Here's how the part is built. I have some questions about the finished solid (model axes, mm). A direction names the side the tool comes from. Round coordinates to 2 decimals unless told otherwise and drop trailing zeros. Order: outer loops, then holes, each group sorted by start corner. A loop starts at its lowest first (then second) coordinate and runs counter-clockwise, first axis right, second up. Notation, with made-up numbers: (50, 22.25) - (89, 22.25) arc R16 ccw to (89, 40.25) - close; hole circle Ø11 at (73, 46.25). An arc over 180 degrees is marked (long way). Answer as a JSON object with one key per item and string values.
```python
from build123d import *

# Parameters (mm, degrees)
BOSS_EXTRUDE1_DEPTH     = 7.14375
SKETCH2_R               = 4.5
CUT_EXTRUDE1_DEPTH      = 31.286531402
CUT_EXTRUDE2_REACH      = 26.287
CUT_EXTRUDE2_END_RADIUS = 4.5
SKETCH3_R               = 4.5


with BuildPart() as part:
    # Sketch1 → Boss-Extrude1 (new, symmetric)
    with BuildSketch(Plane(origin=(0, 0, 0), x_dir=(0, 0, -1), z_dir=(1, 0, 0))):
        Polygon((-13.49375, -7.14375), (13.49375, -7.14375), (13.49375, 7.14375), (7.14375, 7.14375), (7.14375, 11.74375), (-7.14375, 11.74375), (-7.14375, 7.14375), (-13.49375, 7.14375), align=None)
    extrude(amount=BOSS_EXTRUDE1_DEPTH, both=True)

    # Sketch2 → Cut-Extrude1 (cut, through all)
    with BuildSketch(Plane.XY.offset(13.49375)):
        Circle(SKETCH2_R)
    extrude(amount=-CUT_EXTRUDE1_DEPTH, mode=Mode.SUBTRACT)

    # Cut-Extrude2: up to this cylinder (the profile starts outside it)
    cut_extrude2_end = Plane(origin=(0, 0, 0), z_dir=(0, 0, 1)) * Cylinder(CUT_EXTRUDE2_END_RADIUS, 62.574, mode=Mode.PRIVATE)
    # Sketch3 → Cut-Extrude2 (cut, up to the surface)
    with BuildSketch(Plane(origin=(0, 11.74375, 0), x_dir=(1, 0, 0), z_dir=(0, 1, 0)), mode=Mode.PRIVATE) as cut_extrude2_sk1:
        with Locations(Location((0, 0, 0), (0, 0, 270))):
            Circle(SKETCH3_R)
    cut_extrude2_tool1 = extrude(cut_extrude2_sk1.sketch, amount=-CUT_EXTRUDE2_REACH, mode=Mode.PRIVATE) - cut_extrude2_end
    add(cut_extrude2_tool1.solids().sort_by_distance((0, 11.74375, 0))[0], mode=Mode.SUBTRACT)

    # Sketch4 → Cut-Revolve1 (revolve, cut)
    with BuildSketch(Plane(origin=(0, 0, 0), x_dir=(0, 0, -1), z_dir=(0.7071067811865476, 0.7071067811865475, 0))):
        Polygon((13.49375, 10.102788136), (13.99375, 6.967405384), (11.90625, 10.102788136), align=None)
        Polygon((-13.49375, 10.102788136), (-13.99375, 6.967405384), (-11.90625, 10.102788136), align=None)
    revolve(axis=Axis((0, 0, -13.49375), (0, 0, 1)), mode=Mode.SUBTRACT)

    # Sketch5 → Cut-Revolve2 (revolve, cut)
    with BuildSketch(Plane(origin=(0, 0, 0), x_dir=(-0.7071067811865476, 0, -0.7071067811865475), z_dir=(0.7071067811865475, 0, -0.7071067811865476))):
        Polygon((10.102788136, 11.74375), (6.967405384, 12.24375), (10.102788136, 10.15625), align=None)
    revolve(axis=Axis((0, 0, 0), (0, 1, 0)), mode=Mode.SUBTRACT)


solid = part.part
```
1. For faces 1 (the face through (0, 9, -7.144)), 2 (the face through (3.3, 11.744, -3.3)), which set-ups out of +Z, -Z, +X, -X, +Y, -Y let a thin tool reach every point of the face, with its end or its side?
Responses:
{"face 1": "-Z, +X, -X, +Y", "face 2": "+Z, -Z, +X, -X, +Y"}
2. Thinking about a two-plate mould opening in Z: for faces 3 (the face through (5.971, 5.905, -13.042)), 4 (the face through (4.46, 7.26, -0.59)), 5 (the face through (0, 9, 7.144)), which applies, pulls with the +Z half, pulls with the -Z half, needs draft (parallel to the pull), parting line crosses it, or undercut?
Responses:
{"face 3": "pulls with the -Z half", "face 4": "undercut", "face 5": "pulls with the +Z half"}
3. Imagine slicing it at B-B (y = 8). List the corners of the cut face in (x, z) for me, plus the area to 3 significant figures.
Responses:
{"outline": "(-7.14, -7.14) - (7.14, -7.14) - (7.14, 7.14) - (-7.14, 7.14) - close; hole circle Ø9 at (0, 0)", "area": "141 mm2"}
4. If I drill on L1, parallel to X at y = 0, z = -5.25; L2, parallel to Y at x = 0, z = 2.75; L3, parallel to Y at x = 3.75, z = -11, over which ranges is the centre line in solid material (lowest first)? Write a range as [from, to].
Responses:
{"L1": "[-7.14, -4.5], [4.5, 7.14]", "L2": "[-7.14, -4.5]", "L3": "[-7.14, -2.49], [2.49, 7.14]"}
5. For P1, Ø5, axis at x = 3, y = 10, coming from the +Z side; P2, Ø6, axis at x = 3, y = 10, coming from the -Z side; P3, Ø1.9, axis at x = 0.5, z = -10.5, coming from the +Y side; P4, Ø8, axis at x = 0, y = 0, coming from the +Z side, each with a flat end and sliding along its axis, tell me the tip position at first contact or that it passes through.
Responses:
{"P1": "z = 7.14", "P2": "z = -13.49", "P3": "y = 7.14", "P4": "through"}
6. Imagine slicing it at D-D (y = 1). List the corners of the cut face in (x, z) for me.
Responses:
{"outline": "(-7.14, -13.49) - (-4.39, -13.49) - (-4.39, -1) arc R4.5 cw to (-4.39, 1) - (-4.39, 13.49) - (-7.14, 13.49) - close; (4.39, -13.49) - (7.14, -13.49) - (7.14, 13.49) - (4.39, 13.49) - (4.39, 1) arc R4.5 cw to (4.39, -1) - close"}
7. Imagine slicing it at A-A (x = 0). List the corners of the cut face in (y, z) for me, plus the area to 3 significant figures.
Responses:
{"outline": "(-7.14, -13.49) - (-4.5, -13.49) - (-4.5, 13.49) - (-7.14, 13.49) - close; (4.5, -13.49) - (7.14, -13.49) - (7.14, -7.14) - (11.74, -7.14) - (11.74, -4.5) - (4.5, -4.5) - close; (4.5, 4.5) - (11.74, 4.5) - (11.74, 7.14) - (7.14, 7.14) - (7.14, 13.49) - (4.5, 13.49) - close", "area": "143 mm2"}
